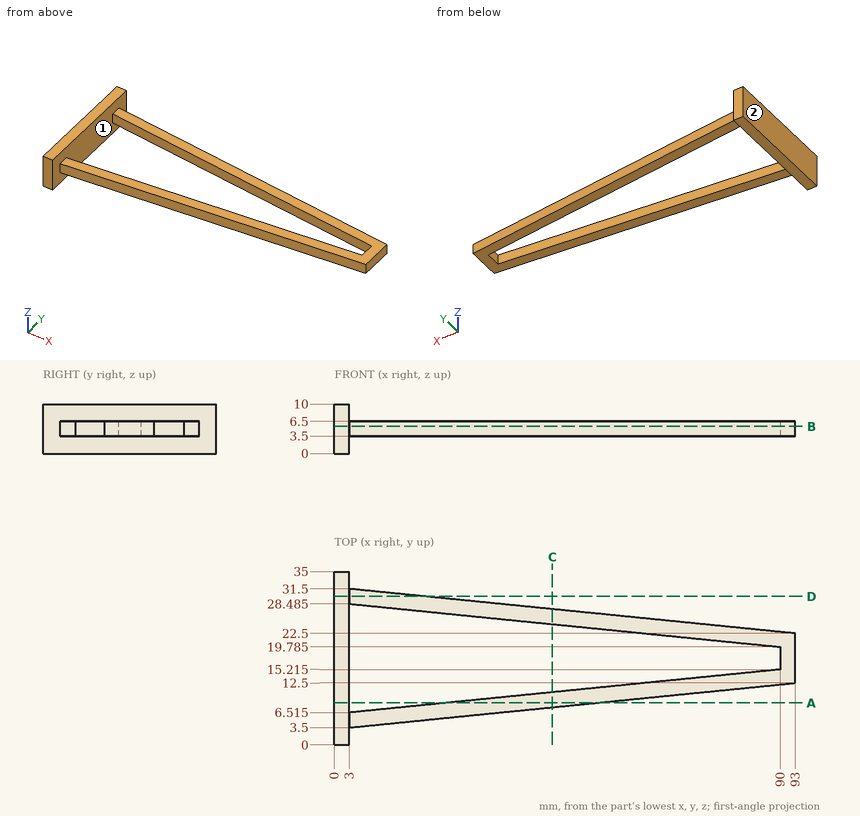
The figure shows three views and two pictorial views of one solid part (mm, origin at its lowest corner). Answer the questions. Coordinates: 2 decimals unless noted, no trailing zeros. Loops run counter-clockwise (first coordinate to the right, second up) from the corner with the lowest first, then second, coordinate; pieces in that order, holes last. Notation, with made-up numbers: (73.5, 22.5) -> (124.5, 22.5) arc R20 cw to (124.5, 58.5) -> close; hole circle Ø10 at (22, 13.25). An arc over 180 degrees is marked (long way). Use one line per item in the form item = value. Start each with the question number.
Item 1: The part is cut by section A-A on y = 8.5. Determine the outline of the cut face in (x, z), then the cut area to 3 significant figures.
Item 2: The part is cut by section D-D on y = 30. Determine the outline of the cut face in (x, z), then the cut area to 3 significant figures.
Item 3: The part is cut by section B-B on z = 5.5. Determine the outline of the cut face in (x, y) (3 decimals).
Item 4: Flat-ended cylindrical pins translate along their axes: pin 1 Ø14 at (x, y) = (42, 14.5) entering from -Z; pin 2 Ø2 at (x, z) = (40.5, 3.5) entering from +Y; pin 3 Ø6 at (x, z) = (73, 1.5) entering from -Y; pin 4 Ø2 at (x, y) = (70, 27.5) entering from +Z. Find the tip coordinate at first contact, or state that the pin passes through.
Item 5: Consider L1, parallel to X at y = 16, z = 3.25; L2, parallel to Y at x = 44.5, z = 4.75 (3 decimals); L3, parallel to Z at x = 69.5, y = 11. Determine where each line is inside the solid, lowest interval first. Write a range as [from, to].
Item 6: The part is cut by section C-C on x = 44. Determine the outline of the cut face in (y, z) (3 decimals), then the cut area to 3 significant figures.
Item 7: The mould has two halves that part along X. Classify the marked faces 1 and 2: released by +X, released by -X, zero draft, split by the parting line, or undercut.
Answer key:
q1.outline = (0, 0) -> (3, 0) -> (3, 10) -> (0, 10) -> close; (22.85, 3.5) -> (53, 3.5) -> (53, 6.5) -> (22.85, 6.5) -> close
q1.area = 120 mm2
q2.outline = (0, 0) -> (3, 0) -> (3, 3.5) -> (18, 3.5) -> (18, 6.5) -> (3, 6.5) -> (3, 10) -> (0, 10) -> close
q2.area = 75.0 mm2
q3.outline = (0, 0) -> (3, 0) -> (3, 3.5) -> (93, 12.5) -> (93, 22.5) -> (3, 31.5) -> (3, 35) -> (0, 35) -> close; hole (3, 6.515) -> (90, 15.215) -> (90, 19.785) -> (3, 28.485) -> close
q4.pin_1 = 3.5
q4.pin_2 = 27.85
q4.pin_3 = 10.28
q4.pin_4 = through
q5.L1 = [0, 3]
q5.L2 = [7.65, 10.665], [24.335, 27.35]
q5.L3 = [3.5, 6.5]
q6.outline = (7.6, 3.5) -> (10.615, 3.5) -> (10.615, 6.5) -> (7.6, 6.5) -> close; (24.385, 3.5) -> (27.4, 3.5) -> (27.4, 6.5) -> (24.385, 6.5) -> close
q6.area = 18.1 mm2
q7.face_1 = undercut
q7.face_2 = released by -X
